For this review, use the dimensioned drawing (mm, ordinates from the lowest corner) and the shaded views. A direction names the side the tool comes from. Round coordinates to 2 decimals unless told otherwise and drop trailing zeros. Order: outer loops, then holes, each group sorted by start corner. A loop starts at its lowest first (then second) coordinate and runs counter-clockwise, first axis right, second up. Notation, with made-up numbers: (-7, 45.5) -> (50, 45.5) arc R11 ccw to (50, 56.5) -> close; hole circle Ø11 at (77.25, 24.25). An arc over 180 degrees is marked (long way). Answer in a Markdown table with one row per item.
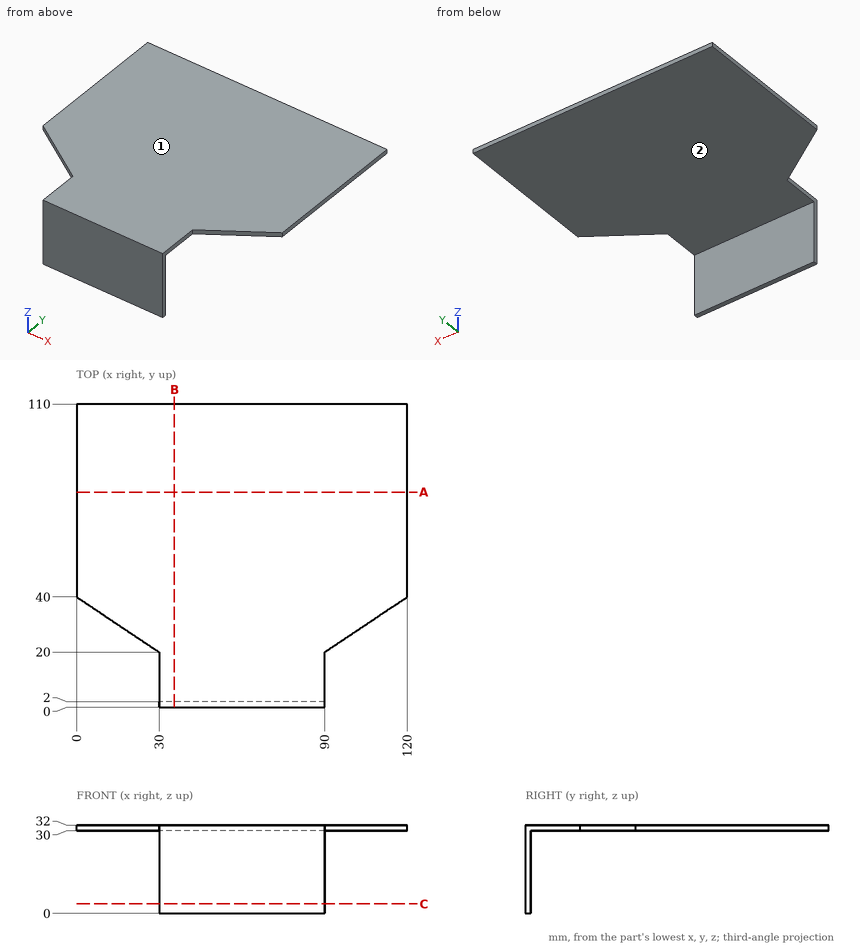
Q1. To check wall thickness, follow probe 1 along Z at (x, y) = (34.5, 102); probe 2 along Y at (x, z) = (80, 27). State the ranges of each line that lie inside material, in increasing order.
Answer key:
| item | result |
|---|---|
| probe 1 | z = 30 to 32 |
| probe 2 | y = 0 to 2 |
Q2. Take a section at B-B, the plane x = 35.5. Write out the cut boundary in (y, z).
Answer key:
| item | result |
|---|---|
| outline | (0, 0) -> (2, 0) -> (2, 30) -> (110, 30) -> (110, 32) -> (0, 32) -> close |
Q3. Take a section at A-A, the plane y = 78. Write out the cut boundary in (x, z), then the cut area to 3 significant figures.
Answer key:
| item | result |
|---|---|
| outline | (0, 30) -> (120, 30) -> (120, 32) -> (0, 32) -> close |
| area | 240 mm^2 |
Q4. Tool access review of the marked faces 1 and 2: name each direction out of +Z, -Z, +X, -X, +Y, -Y from which nothing blocks a thin tool from reaching the whole face with its end or side.
Answer key:
| item | result |
|---|---|
| face 1 | +Z, +X, -X, +Y, -Y |
| face 2 | -Z, +X, -X, +Y |
Q5. Take a section at C-C, the plane z = 3.5. Write out the cut boundary in (x, y), then the cut area to 3 significant figures.
Answer key:
| item | result |
|---|---|
| outline | (30, 0) -> (90, 0) -> (90, 2) -> (30, 2) -> close |
| area | 120 mm^2 |
Q6. Clearance check with flat-ended pins moving along their axes: pin 1 Ø9 at (x, z) = (52, 12) entering from +Y; pin 2 Ø3 at (x, y) = (79, 92.5) entering from -Z. State where each tip first meets the part, or that it passes through.
Answer key:
| item | result |
|---|---|
| pin 1 | stops at y = 2 |
| pin 2 | stops at z = 30 |
